Design review of the part shown in the three views and the two pictorial views. Dimensions are in mm from the part's minimum x, y and z. A direction names the side the tool comes from. Round coordinates to 2 decimals unless told otherwise and drop trailing zeros. Order: outer loops, then holes, each group sorted by start corner. A loop starts at its lowest first (then second) coordinate and runs counter-clockwise, first axis right, second up. Notation, with made-up numbers: (-26.5, 82) - (19.5, 82) arc R4 cw to (19.5, 86) - close; hole circle Ø7 at (13, 54). An arc over 180 degrees is marked (long way). One line per question, with ' | ' between items. Start each with the question number.
Item 1: For L1, parallel to X at y = 6, z = 0.3; L2, parallel to Z at x = 17.4, y = 6; L3, parallel to Y at x = 6, z = 0.2, list the stretches that pass through material, from the lowest coordinate up. Write a range as [from, to].
Item 2: Draft analysis for pull direction Y (two halves, no side actions). For the marked faces 3, 4 and 5, state which applies: +Y half, -Y half, draft (parallel to the pull), parting line (faces both ways), or undercut.
Item 3: Insertion check: pin 1 Ø1 at (y, z) = (2, 1.5) entering from +X; pin 2 Ø1.9 at (x, z) = (18.5, 0.5) entering from -Y; pin 3 Ø0.8 at (y, z) = (6, 2.5) entering from -X; pin 4 Ø1 at (y, z) = (5, 0.5) entering from -X. Each pin has a flat end and moves straight along its axis. Give the tip position at first contact, or say it passes through.
Item 4: Add section B-B on z = 1.3. State the section outline as (x, y) points.
Item 5: Add section D-D on x = 2.25. State the section outline as (y, z) points.
Item 6: Add section C-C on y = 7.25. State the section outline as (x, z) points.
Item 7: Tool access review of the marked faces 1 and 2: name each direction out of +Z, -Z, +X, -X, +Y, -Y from which nothing blocks a thin tool from reaching the whole face with its end or side.
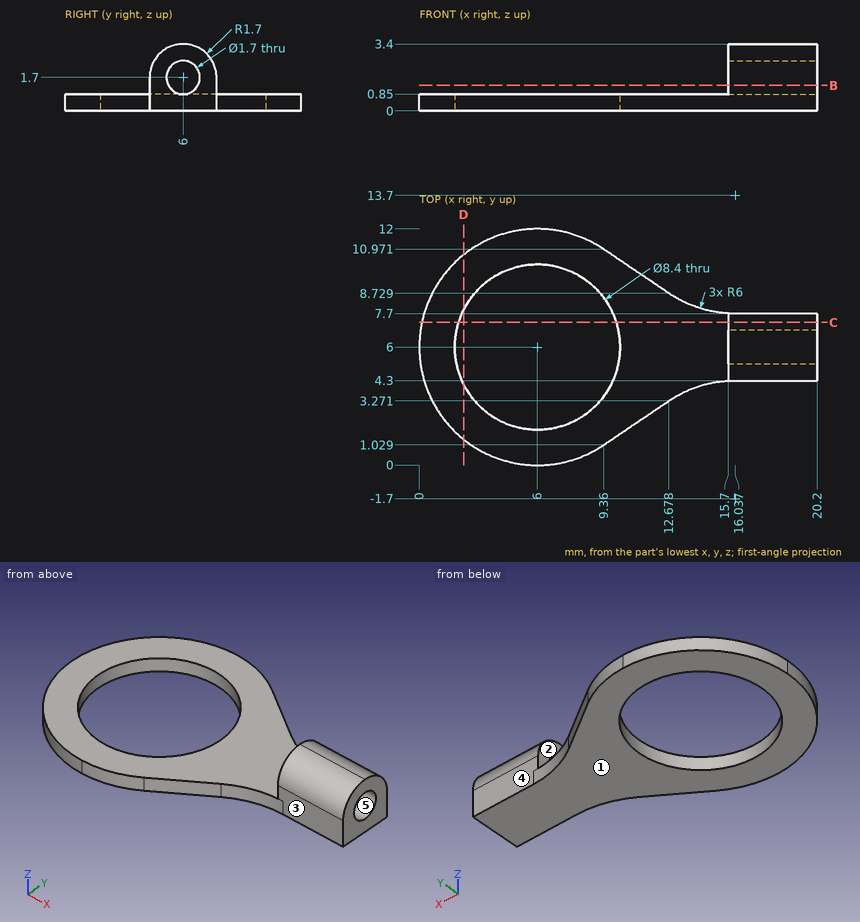
Determined:
1) L1: [0, 1.8], [10.2, 20.2] | L2: [0, 0.85], [2.55, 3.4] | L3: [0, 1.8], [10.2, 12]
2) face 3: -Y half | face 4: +Y half | face 5: undercut
3) pin 1: through | pin 2: y = 4.3 | pin 3: x = 15.7 | pin 4: x = 0.02
4) outline: (15.7, 4.3) - (20.2, 4.3) - (20.2, 5.25) - (15.7, 5.25) - close; (15.7, 6.75) - (20.2, 6.75) - (20.2, 7.7) - (15.7, 7.7) - close
5) outline: (1.32, 0) - (4.11, 0) - (4.11, 0.85) - (1.32, 0.85) - close; (7.89, 0) - (10.68, 0) - (10.68, 0.85) - (7.89, 0.85) - close
6) outline: (0.13, 0) - (1.99, 0) - (1.99, 0.85) - (0.13, 0.85) - close; (10.01, 0) - (20.2, 0) - (20.2, 2.85) - (15.7, 2.85) - (15.7, 0.85) - (10.01, 0.85) - close
7) face 1: -Z, +X, -X, +Y, -Y | face 2: +Z, -X, +Y, -Y
